Check sheet for the modelled part. Datum: model origin and axes. Units: mm. A direction names the side the tool comes from. Give positions to 0.01 mm unless a question says otherwise; leave off trailing zeros. Loops run counter-clockwise (first coordinate to the right, second up) from the corner with the lowest first, then second, coordinate; pieces in that order, holes last. Notation, with made-up numbers: (76, 63) -> (106, 63) arc R36 ccw to (106, 99) -> close; hole circle Ø5 at (15.5, -28.5). An arc over 180 degrees is marked (long way). Write each question's results on one line, items separated by ' | '. Start each with the question number.
Item 1: Scan lines: line 1 along X through (y, z) = (-3, -4.5); line 2 along Y through (x, z) = (-2, 3); line 3 along Y through (x, z) = (-3.5, -1). Record each from-to range of solid material in increasing order.
Item 2: Cross-section at A-A on x = 2.5. Enter the section's corners in (y, z), then the cut area to 3 significant figures.
Item 3: Mould release check, pull along Z, two halves, no side actions. Record for faces 4 (the face through (5, -3, 0)), 5 (the face through (-3, 0, -1.289)), 6 (the face through (10, 0, 0)): pulls with the +Z half, pulls with the -Z half, needs draft (parallel to the pull), parting line crosses it, or undercut.
Item 4: Gauge pin test, flat ends, axial feed: pin 1 Ø2.5 at (x, z) = (-3, 0) entering from +Y; pin 2 Ø4 at (x, z) = (7.5, 0) entering from -Y; pin 3 Ø0.7 at (x, z) = (-3, 0.5) entering from -Y; pin 4 Ø0.7 at (x, y) = (-2.5, -0.5) entering from -Z. Record the tip position at first contact, or that the pin passes through.
Item 5: Access from +Z, -Z, +X, -X, +Y, -Y to the whole of each face (thin tool, end or side, straight path). Record for faces 1 (the face through (-1, -6, 0)), 2 (the face through (-1.151, -1.064, 0.018)), 3 (the face through (0, 3, -3)).
Autodesk Inventor part; units mm, degrees
ref_plane "IDS_WORKPLANE{1}" through (-4.6, 0, 0) normal (1, 0, 0) x (0, 0, -1)
ref_plane "Work Plane2" through (69.85, 0, 0) normal (0, 0, -1) x (1, 0, 0)
ref_plane "YZ Plane" through (0, 0, 0) normal (1, 0, 0) x (0, 1, 0)
sketch "Sketch1" plane through (0, 0, 0) normal (0, 0, 1) x (1, 0, 0)
  line L0 (-0.59, 0) -> (10, 0)
  line L1 (10, 0) -> (10, 3)
  line L2 (10, 3) -> (0, 3)
  line L3 (0, 3) -> (0, 6)
  line L4 (-8.1003, 0) -> (13.0167, 0)
  line L5 (0, -1.2172) -> (0, 7.3031)
  line L6 (-4.6, 2.3998) -> (-5.0836, 2.3998) construction
  line L7 (-4.6, 0) -> (-0.59, 0)
  line L8 (0, 0) -> (-0.59, 0)
  line L9 (-4.6, 0) -> (-4.6, 6)
  arc A0 (-2.8922, 6) -> (-4.6, 2.3998) centre (5.1078, 0) ccw
  line L10 (-4.6, 6) -> (0, 6)
  dimension "d0" = 10
  dimension "d1" = 6
  dimension "d2" = 12
  dimension "d4" = 4.7996
  dimension "d13" = 4.6
  dimension "d14" = 4.01
  dimension "d46" = 10
  dimension "d47" = 0
revolve "Body" add sketch "Sketch1" angle 360 about axis through (-0.59, 0, 0) along (1, 0, 0) contours L4 L9 A0 L10 L3 L5 L0 | L5 L2 L1 L0
ref_plane "IDS_WORKPLANE{1}" through (-4.6, 0, 0) normal (1, 0, 0) x (0, 0, -1)
sketch "Sketch2" plane through (-4.6, 0, 0) normal (1, 0, 0) x (0, 0, -1)
  line L0 (0, -8.4) -> (0, 8.4)
  line L1 (8.4, 0) -> (-8.4, 0)
  line L2 (-1.289, 1.289) -> (1.289, 1.289)
  line L3 (1.289, 1.289) -> (1.289, -1.289)
  line L4 (1.289, -1.289) -> (-1.289, -1.289)
  line L5 (-1.289, -1.289) -> (-1.289, 1.289)
  line L6 (0, 1.289) -> (0, -1.289) construction
  line L7 (-1.289, 0) -> (1.289, 0) construction
  dimension "d7" = 2.578
  dimension "d9" = 2.578
extrude "Extrusion" cut sketch "Sketch2" along normal blind 4.01
fillet "Fillet1" radius 1.289 4 edges at (-0.59, 0, -1.289) (-0.59, -1.289, 0) (-0.59, 0, 1.289) (-0.59, 1.289, 0)
chamfer "Chamfer1" distance 0.401 angle 45 4 edges at (-4.6, 1.289, 0) (-4.6, 0, -1.289) (-4.6, -1.289, 0) (-4.6, 0, 1.289)
thread "Thread"
chamfer "Chamfer2" distance 0.875 distance2 0.6135 1 edges at (10, -3, 0) measured on face at (10, 0.705, 0.3049)
ref_plane "Work Plane2" through (69.85, 0, 0) normal (0, 0, -1) x (1, 0, 0)
fillet "Fillet2" radius 0.3 1 edges at (0, -3, 0)
equation "\"d0\" = NLG"
equation "\"d1\" = GD"
equation "\"d2\" = KOD"
equation "\"d4\" = 1.42 * KOM"
equation "\"d13\" = KOH"
equation "\"d14\" = STI"
equation "\"d46\" = KR"
equation "\"d7\" = KOM - 0.2 * STI"
equation "\"d9\" = KOM - 0.2 * STI"
equation "\"d48\" = STI"
equation "\"d50\" = -0.1 * STI + 0.5 * KOM"
equation "\"d51\" = 0.1 * STI"
equation "\"d18\" = GEL"
equation "\"d20\" = -0.5 * SPD + 0.5 * GD"
equation "\"d21\" = GUL"
equation "\"d44\" = R"
equation "\"GD\" = 6"
equation "\"NLG\" = 10"
equation "\"GEL\" = 9"
equation "\"KOD\" = 12"
equation "\"KOH\" = 4.6"
equation "\"SPD\" = 4.25"
equation "\"KR\" = 10"
equation "\"RR\" = 2"
equation "\"GUL\" = 0.61345 * PTC"
equation "\"KEWI\" = 0"
equation "\"SDM\" = 3.38"
equation "\"STI\" = 4.01"
equation "\"d6\" = -KOH"
equation "\"R\" = 0.3"
equation "\"KOM\" = 3.38"
equation "\"PTC\" = 1"
properties part number "ANSI B18.6.7M - M6x1 x 10, SRPHMSTIM" material "Steel, Mild"
Answer sheet:
1) line 1: x = -3.3 to 0 | line 2: y = -5.2 to 5.2 | line 3: y = -4.99 to -1.29, 1.29 to 4.99
2) outline: circle Ø6 at (0, 0) | area: 28.3 mm²
3) face 4: parting line crosses it | face 5: undercut | face 6: needs draft
4) pin 1: stops at y = 6 | pin 2: stops at y = -3 | pin 3: stops at y = -6 | pin 4: stops at z = -6
5) face 1: +X, -X | face 2: -X | face 3: +X
